The listing builds one solid part. Answer for the finished solid, in the listing's coordinates (mm). A direction names the side the tool comes from. Give positions to 0.01 mm unless a question says otherwise; leave off trailing zeros. Write each loop counter-clockwise with the first axis right and the second up, starting at its lowest first coordinate (ties: lowest second). Pieces come first, ordered by that corner, then holes. Notation, with made-up numbers: M 25,-20 L 51,-20 A30 ccw 51,16 Z; hole C -26,-10.5 d3. An arc over 180 degrees is marked long. Answer as a JSON object with one key per item and string values.
Autodesk Inventor part; units mm, degrees
ref_plane "作業平面5" through (0, -6, 90) normal (0, -1, 0) x (1, 0, 0)
ref_plane "YZ Plane" through (0, 0, 0) normal (1, 0, 0) x (0, 1, 0)
ref_plane "XZ Plane" through (0, 0, 0) normal (0, 1, 0) x (-1, 0, 0)
sketch "スケッチ1" plane through (0, 0, 0) normal (0, 0, 1) x (1, 0, 0)
  circle A0 centre (0, 0) radius 6
  dimension "d0" = 12
extrude "押し出し1" add sketch "スケッチ1" along normal blind 35
thread "ねじ1"
sketch "スケッチ2" plane through (0, 0, 35) normal (0, 0, 1) x (1, 0, 0)
  circle A0 centre (0, 0) radius 6
  dimension "d5" = 12
extrude "押し出し2" add sketch "スケッチ2" along normal blind 55
sketch "スケッチ6" plane through (0, 0, 90) normal (0, 0, 1) x (1, 0, 0)
  line L0 (0, 0) -> (0, -6) construction
  circle A0 centre (0, 0) radius 6
ref_plane "作業平面5" through (0, -6, 90) normal (0, -1, 0) x (1, 0, 0)
sketch "スケッチ8" plane through (0, -6, 90) normal (0, -1, 0) x (1, 0, 0)
  line L0 (6, 0) -> (-6, 0)
  line L1 (-2, 0) -> (2, 0)
  line L2 (-2, 0) -> (2, 0)
  line L3 (2, 0) -> (2, -48)
  line L4 (-2, -48) -> (-2, 0)
  arc A0 (-2, -48) -> (2, -48) centre (0, -48) ccw
  point P0 (0, -90)
  point P1 (0, 0)
  dimension "d11" = 2
  dimension "d17" = 48
  dimension "d29" = 2
extrude "押し出し3" cut sketch "スケッチ8" against normal blind 2.157
sketch "スケッチ9" plane through (0, 0, 90) normal (0, 0, 1) x (1, 0, 0)
  point P0 (0, 0)
  point P1 (0, 0)
hole "穴1" at (0, 0, 90) direction (0, 0, -1) diameter 5 depth 8 tip angle 118
thread "ねじ2"
thread "ねじ3"
properties part number "正しい"
1. Flat-ended cylindrical pins translate along their axes: pin 1 (6 mm diameter, centred on x = -4.5, z = 14, fed in from -Y); pin 2 (2 mm diameter, centred on x = 0.5, z = 68.5, fed in from -Y); pin 3 (1.5 mm diameter, centred on y = -4.5, z = 58, fed in from +X). Find the tip coordinate at first contact, or state that the pin passes through.
Verdict:
{"pin 1": "stops at y = -5.81", "pin 2": "stops at y = -3.84", "pin 3": "stops at x = 4.68"}
2. A cutting plane is placed at A-A, the plane z = 68. Give the vertices of the cut face in (x, y).
Verdict:
{"outline": "M -2,-5.66 L -2,-3.84 L 2,-3.84 L 2,-5.66 A6 ccw long Z"}
3. The mould has two halves that part along Y. Classify faces 1 (the conical face through (-0.424, 0.094, 80.759)), 2 (the flat face through (2, -5, 66)), 3 (the cylindrical face through (-1.301, 5.857, 44.37)), 4 (the cylindrical face through (2.44, 0.54, 85.94)): released by +Y, released by -Y, zero draft, split by the parting line, or undercut.
Verdict:
{"face 1": "undercut", "face 2": "zero draft", "face 3": "split by the parting line", "face 4": "undercut"}
4. A cutting plane is placed at C-C, the plane y = 4.25. Give the vertices of the cut face in (x, z), plus the area to 3 significant figures.
Verdict:
{"outline": "M -4.24,0 L 4.24,0 L 4.24,90 L -4.24,90 Z", "area": "762 mm2"}
5. A cutting plane is placed at B-B, the plane z = 36. Give the vertices of the cut face in (x, y), plus the area to 3 significant figures.
Verdict:
{"outline": "C 0,0 d12", "area": "113 mm2"}
6. For faces 5 (the flat face through (0, 3, 90)), 6 (the flat face through (-2, -5, 66)), determine the directions among +Z, -Z, +X, -X, +Y, -Y from which every point of the face is accessible in a straight line to the end or side of a thin tool.
Verdict:
{"face 5": "+Z, +X, -X, +Y, -Y", "face 6": "+Z, -Y"}
7. Consider line 1 along Y through (x, z) = (0, 87.25); line 2 along X through (y, z) = (0, 87.5); line 3 along X through (y, z) = (-1.25, 83.5). Determine where each line is inside the solid, lowest interval first.
Verdict:
{"line 1": "y = -3.84 to -2.5, 2.5 to 6", "line 2": "x = -6 to -2.5, 2.5 to 6", "line 3": "x = -5.87 to -2.17, 2.17 to 5.87"}
